```python
from build123d import *

# Parameters (mm, degrees)
F0_W     = 304.8
F0_H     = 203.2
F0_R     = 6.35
F1_DEPTH = 12
F3_D     = 5


with BuildPart() as f1:
    # F0 (on Top) → F1 (new body)
    with BuildSketch(Plane.XY):
        with Locations((-4.632816, 0.599919)):
            Rectangle(F0_W, F0_H)
        with Locations((119.592541, -84.271215)):
            Circle(F0_R, mode=Mode.SUBTRACT)
        with Locations((50.8, -44.45)):
            Circle(F0_R, mode=Mode.SUBTRACT)
        with Locations((50.8, -30.264465)):
            Circle(F0_R, mode=Mode.SUBTRACT)
        with Locations((-50.8, 30.48)):
            Circle(F0_R, mode=Mode.SUBTRACT)
        with Locations((-50.8, 44.45)):
            Circle(F0_R, mode=Mode.SUBTRACT)
        with Locations((-135.430858, 83.075233)):
            Circle(F0_R, mode=Mode.SUBTRACT)
    extrude(amount=-F1_DEPTH)

    # F3 (through all)
    with Locations(Plane.XY):
        with Locations((0, 0)):
            Hole(F3_D / 2)


solid = f1.part
```
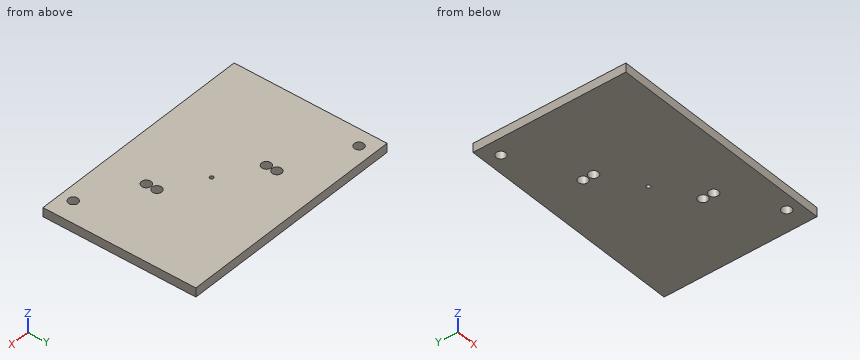
Here's how the part is built. I have some questions about the finished solid (model axes, mm). Give positions to 0.01 mm unless a question says otherwise; leave off trailing zeros. Write each loop counter-clockwise with the first axis right and the second up, starting at its lowest first coordinate (ties: lowest second). Pieces come first, ordered by that corner, then holes.
(1) If I drill on L1, parallel to Y at x = 50.8, z = -6.5; L2, parallel to Y at x = 0, z = -3; L3, parallel to Y at x = -135.5, z = -2.5, over which ranges is the centre line in solid material (lowest first)?
Output values:
L1: y = -101 to -50.8, -38.1 to -36.61, -23.91 to 102.2
L2: y = -101 to -2.5, 2.5 to 102.2
L3: y = -101 to 76.73, 89.42 to 102.2
(2) Imagine slicing it at C-C, the plane y = -27. Write out the boundary of the cut face in (x, z), and give its area (3 significant figures).
Output values:
outline: (-157.03, -12) - (45.35, -12) - (45.35, 0) - (-157.03, 0) - close; (56.25, -12) - (147.77, -12) - (147.77, 0) - (56.25, 0) - close
area: 3,530 mm2
(3) Imagine slicing it at B-B, the plane y = 44.45. Write out the boundary of the cut face in (x, z), and give its area (3 significant figures).
Output values:
outline: (-157.03, -12) - (-57.15, -12) - (-57.15, 0) - (-157.03, 0) - close; (-44.45, -12) - (147.77, -12) - (147.77, 0) - (-44.45, 0) - close
area: 3,510 mm2
(4) Imagine slicing it at A-A, the plane x = 50.8. Write out the boundary of the cut face in (y, z).
Output values:
outline: (-101, -12) - (-50.8, -12) - (-50.8, 0) - (-101, 0) - close; (-38.1, -12) - (-36.61, -12) - (-36.61, 0) - (-38.1, 0) - close; (-23.91, -12) - (102.2, -12) - (102.2, 0) - (-23.91, 0) - close
